Can you work these out from the drawing? Everything is in mm from the part's minimum corner. A direction names the side the tool comes from. Give positions to 0.01 mm unless a question says otherwise; leave off trailing zeros. Write each loop counter-clockwise with the first axis right and the second up, starting at its lowest first coordinate (ties: lowest second). Pieces come first, ordered by that corner, then holes. Notation, with made-up numbers: (26.25, 44.5) -> (55.25, 44.5) arc R37 ccw to (55.25, 81.5) -> close; hole circle Ø7 at (-4.5, 30). An arc over 180 degrees is marked (long way). Return JSON: item names as keys, results as strings.
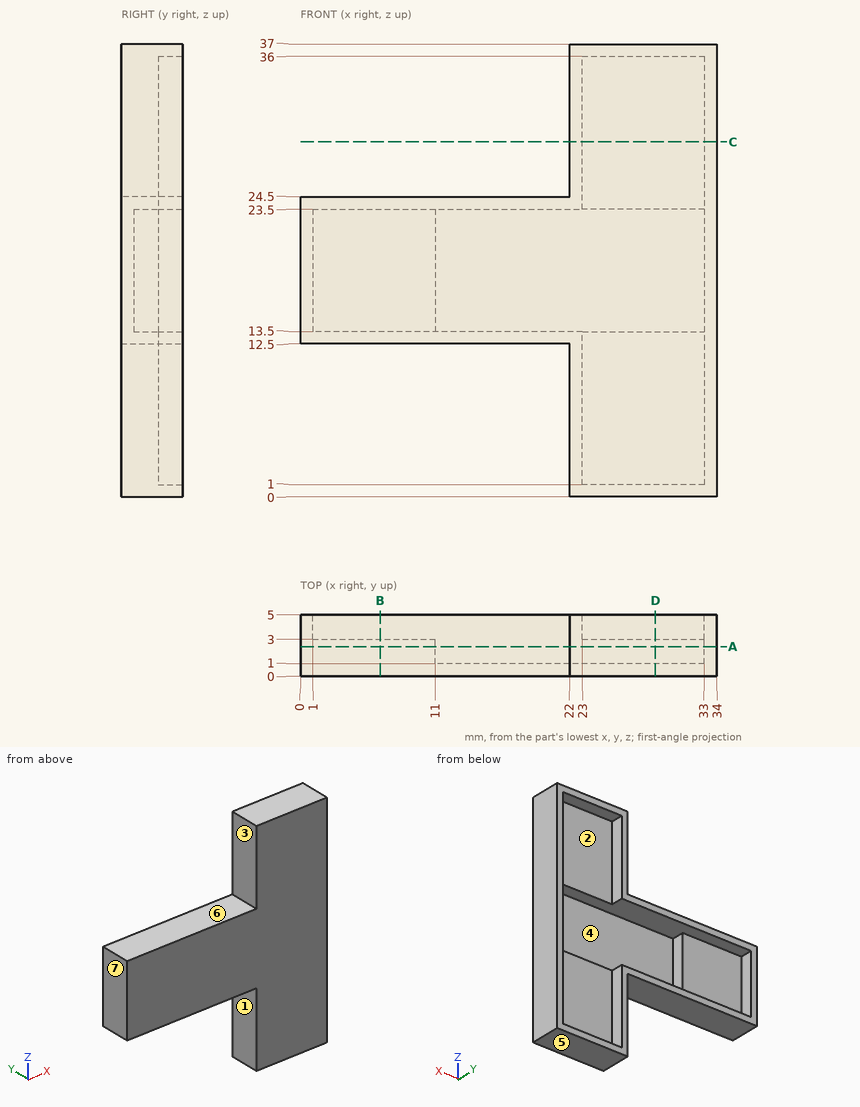
1. Suppose I cut it at D-D, the plane x = 29. List the corners of the cut face in (y, z) for me.
Taken from the geometry:
{"outline": "(0, 0) -> (5, 0) -> (5, 1) -> (3, 1) -> (3, 13.5) -> (1, 13.5) -> (1, 23.5) -> (3, 23.5) -> (3, 36) -> (5, 36) -> (5, 37) -> (0, 37) -> close"}
2. Suppose I cut it at C-C, the plane z = 29. List the corners of the cut face in (x, y) for me.
Taken from the geometry:
{"outline": "(22, 0) -> (34, 0) -> (34, 5) -> (33, 5) -> (33, 3) -> (23, 3) -> (23, 5) -> (22, 5) -> close"}
3. Suppose I cut it at A-A, the plane y = 2.4. List the corners of the cut face in (x, z) for me.
Taken from the geometry:
{"outline": "(0, 12.5) -> (22, 12.5) -> (22, 0) -> (34, 0) -> (34, 37) -> (22, 37) -> (22, 24.5) -> (0, 24.5) -> close; hole (11, 13.5) -> (33, 13.5) -> (33, 23.5) -> (11, 23.5) -> close"}
4. Suppose I cut it at B-B, the plane x = 6.5. List the corners of the cut face in (y, z) for me.
Taken from the geometry:
{"outline": "(0, 12.5) -> (5, 12.5) -> (5, 13.5) -> (3, 13.5) -> (3, 23.5) -> (5, 23.5) -> (5, 24.5) -> (0, 24.5) -> close"}
5. For pin 1 Ø3 at (y, z) = (1, 10.5) entering from -X; pin 2 Ø1 at (x, z) = (6, 16.5) entering from +Y; pin 3 Ø2 at (x, y) = (9, 2) entering from +Z; pin 4 Ø8 at (x, z) = (26.5, 8) entering from +Y, each with a flat end and sliding along its axis, tell me the tip position at first contact or that it passes through.
Taken from the geometry:
{"pin 1": "stops at x = 22", "pin 2": "stops at y = 3", "pin 3": "stops at z = 24.5", "pin 4": "stops at y = 5"}
6. Which directions (+Z, -Z, +X, -X, +Y, -Y) give clear straight access to the entire face, cutting with the end or side of a thin tool? Please do the marked faces 1, 2 and 3.
Taken from the geometry:
{"face 1": "-Z, -X, +Y, -Y", "face 2": "+Y", "face 3": "+Z, -X, +Y, -Y"}
7. If I drill on line 1 (X direction, y = 3.3, z = 31.5); line 2 (Z direction, x = 9.5, y = 3.4); line 3 (X direction, y = 1.4, z = 16.5), over which ranges is the centre line in solid material (lowest first)? Write a range as [from, to].
Taken from the geometry:
{"line 1": "x = [22, 23], [33, 34]", "line 2": "z = [12.5, 13.5], [23.5, 24.5]", "line 3": "x = [0, 11], [33, 34]"}
8. If we mould it in two halves opening along Z, with no side actions, what happens to the marked faces 4, 5, 6 and 7? For each: released by +Z, released by -Z, zero draft, split by the parting line, or undercut.
Taken from the geometry:
{"face 4": "undercut", "face 5": "released by -Z", "face 6": "released by +Z", "face 7": "zero draft"}
